Read the model definition and answer for the solid it produces. Units are mm, in the model's axes. A direction names the side the tool comes from. Coordinates: 2 decimals unless noted, no trailing zeros. Write each loop counter-clockwise with the first axis right and the second up, starting at its lowest first coordinate (ties: lowest second). Pieces come first, ordered by that corner, then holes.
(1) Which of the six approach directions +Z, -Z, +X, -X, +Y, -Y give full straight-line access (tool end or side, diameter ignored) to faces 1 (the cylindrical face through (-28.6, 7.54, 18.43)), 2 (the flat face through (-18, 3, 14)), 3 (the cylindrical face through (-11.57, 7.54, 28.6))?
(2) The part is cut by section D-D, the plane x = -14.5. Determine the outline of the cut face in (y, z), and give its area (3 significant figures).
(3) Straight lines are drawn through the part: line 1 along Z through (x, y) = (-3.7, 2.45); line 2 along X through (y, z) = (1.95, 3.7); line 3 along X through (y, z) = (3.75, 4.75). For each, find the intervals that lie inside material, in ascending order.
(4) Given pin 1 (10 mm diameter, centred on x = -19, z = 17, fed in from +Y); pin 2 (3 mm diameter, centred on x = -3.7, z = 26.3, fed in from -Y); pin 3 (2.5 mm diameter, centred on x = -15.5, z = 17.5, fed in from -Y), each flat-ended and moving along its own axis, determine where each tip first touches the part or whether it passes through.
(5) The part is cut by section B-B, the plane z = 15. Determine the outline of the cut face in (x, y).
(6) Determine the mould class of faces 4 (the cylindrical face through (-0.6, 2.54, 29.43)), 5 (the cylindrical face through (-28.57, 7.54, 11.6)), 6 (the flat face through (-12.997, 1.479, 11.595)) for opening direction Z: pulls with the +Z half, pulls with the -Z half, needs draft (parallel to the pull), parting line crosses it, or undercut.
(7) The part is cut by section A-A, the plane y = 6.25. State how many separate pieces and enclosed holes the cut face has, and give its area (3 significant figures).
(8) The part is cut by section C-C, the plane z = 26.3. Determine the outline of the cut face in (x, y).
Autodesk Inventor part; units mm, degrees
ref_plane "YZ Plane" through (0, 0, 0) normal (1, 0, 0) x (0, 1, 0)
ref_plane "XZ Plane" through (0, 0, 0) normal (0, 1, 0) x (-1, 0, 0)
ref_plane "XY Plane" through (0, 0, 0) normal (0, 0, 1) x (1, 0, 0)
sketch "Skizze1" plane through (0, 0, 0) normal (0, 1, 0) x (-1, 0, 0)
  line L0 (0, 0) -> (30, 0)
  line L1 (30, 0) -> (30, 30)
  line L2 (30, 30) -> (0, 30)
  line L3 (0, 30) -> (0, 0)
  dimension "d0" = 30
  dimension "d1" = 30
extrude "Extrusion1" add sketch "Skizze1" along normal blind 5
sketch "Skizze2" plane through (0, 5, 0) normal (0, 1, 0) x (1, 0, 0)
  line L0 (-30, -19) -> (-28, -19)
  line L1 (-28, -19) -> (-28, -11)
  line L2 (-28, -11) -> (-30, -11)
  line L3 (-30, -11) -> (-30, -19)
  line L4 (-19, -2) -> (-11, -2)
  line L5 (-11, -2) -> (-11, 0)
  line L6 (-11, 0) -> (-19, 0)
  line L7 (-19, 0) -> (-19, -2)
  line L8 (-2, -19) -> (0, -19)
  line L9 (0, -19) -> (0, -11)
  line L10 (0, -11) -> (-2, -11)
  line L11 (-2, -11) -> (-2, -19)
  line L12 (-19, -30) -> (-11, -30)
  line L13 (-11, -30) -> (-11, -28)
  line L14 (-11, -28) -> (-19, -28)
  line L15 (-19, -28) -> (-19, -30)
  line L16 (-30, 0) -> (-30, -30)
  line L17 (0, 0) -> (-30, 0)
  line L18 (0, -30) -> (0, 0)
  line L19 (-30, -30) -> (0, -30)
  dimension "d4" = 0
  dimension "d5" = 0
  dimension "d6" = 0
  dimension "d7" = 0
  dimension "d8" = 2
  dimension "d9" = 8
  dimension "d10" = 11
  dimension "d11" = 11
  dimension "d12" = 11
extrude "Extrusion2" add sketch "Skizze2" along normal blind 5 contours L3 L2 L1 L0 | L15 L14 L13 L12 | L6 L5 L4 L7 | L8 L11 L10 L9
sketch "Skizze3" plane through (0, 5, 0) normal (0, 1, 0) x (1, 0, 0)
  line L0 (0, -30) -> (0, -19)
  line L1 (-11, -30) -> (0, -30)
  line L2 (0, 0) -> (-11, 0)
  line L3 (0, -11) -> (0, 0)
  line L4 (-30, -19) -> (-30, -30)
  line L5 (-30, -30) -> (-19, -30)
  line L6 (-30, 0) -> (-30, -11)
  line L7 (-19, 0) -> (-30, 0)
  point P0 (-26.3, -26.3)
  point P1 (-26.3, -3.7)
  point P2 (-3.7, -3.7)
  point P3 (-3.7, -26.3)
  dimension "d15" = 3.7
  dimension "d16" = 3.7
  dimension "d17" = 3.7
  dimension "d18" = 3.7
  dimension "d19" = 3.7
  dimension "d20" = 3.7
  dimension "d21" = 3.7
  dimension "d22" = 3.7
hole "Bohrung1" at (-26.3, 5, 26.3) at (-26.3, 5, 3.7) at (-3.7, 5, 3.7) at (-3.7, 5, 26.3) direction (0, -1, 0) diameter 3.4 end through all
sketch "Skizze4" plane through (0, 5, 0) normal (0, 1, 0) x (1, 0, 0)
  line L0 (-19, 0) -> (-30, 0)
  line L1 (0, -11) -> (0, 0)
  point P0 (-15, -15)
  dimension "d30" = 15
  dimension "d31" = 15
hole "Bohrung2" at (-15, 5, 15) direction (0, -1, 0) diameter 5.5 end through all
sketch "Skizze6" plane through (0, 0, 0) normal (0, -1, 0) x (1, 0, 0)
  line L0 (0, 0) -> (-30, 0)
  line L1 (0, 30) -> (0, 0)
  line L2 (-11.05, 17.2805) -> (-11.05, 12.7195)
  line L3 (-11.05, 12.7195) -> (-15, 10.4389)
  line L4 (-15, 10.4389) -> (-18.95, 12.7195)
  line L5 (-18.95, 12.7195) -> (-18.95, 17.2805)
  line L6 (-18.95, 17.2805) -> (-15, 19.5611)
  line L7 (-15, 19.5611) -> (-11.05, 17.2805)
  point P0 (-15, 15)
  point P1 (-15, 15)
  dimension "d41" = 15
  dimension "d42" = 15
  dimension "d43" = 7.9
extrude "Extrusion3" cut sketch "Skizze6" against normal blind 3
fillet "Rundung1" radius 2 12 edges at (-30, 2.5, 0) (0, 2.5, 0) (-30, 2.5, 30) (0, 2.5, 30) (-11, 7.5, 28) (-19, 7.5, 28) (-28, 7.5, 19) (-28, 7.5, 11) (-2, 7.5, 19) (-2, 7.5, 11) (-19, 7.5, 2) (-11, 7.5, 2)
properties part number "feet_screw_adapter"
Computed:
1. face 1: +Z, +Y
1. face 2: -Y
1. face 3: +X, +Y
2. outline: (0, 0) - (10, 0) - (10, 2) - (5, 2) - (5, 12.3) - (3, 12.3) - (3, 10.73) - (0, 10.73) - close; (0, 19.27) - (3, 19.27) - (3, 17.7) - (5, 17.7) - (5, 28) - (10, 28) - (10, 30) - (0, 30) - close
2. area: 134 mm2
3. line 1: z = 0 to 2, 5.4 to 24.6, 28 to 30
3. line 2: x = -30 to -28, -24.6 to -5.4, -2 to 0
3. line 3: x = -30 to -27.64, -24.96 to -5.04, -2.36 to 0
4. pin 1: stops at y = 5
4. pin 2: passes through
4. pin 3: stops at y = 3
5. outline: (-30, 0) - (-18.95, 0) - (-18.95, 3) - (-17.75, 3) - (-17.75, 5) - (-28, 5) - (-28, 10) - (-30, 10) - close; (-12.25, 3) - (-11.05, 3) - (-11.05, 0) - (0, 0) - (0, 10) - (-2, 10) - (-2, 5) - (-12.25, 5) - close
6. face 4: pulls with the +Z half
6. face 5: pulls with the -Z half
6. face 6: undercut
7. separate pieces: 4
7. enclosed holes: 0
7. area: 57.1 mm2
8. outline: (-30, 0) - (-28, 0) - (-28, 5) - (-30, 5) - close; (-24.6, 0) - (-5.4, 0) - (-5.4, 5) - (-24.6, 5) - close; (-2, 0) - (0, 0) - (0, 5) - (-2, 5) - close
